Autodesk Inventor part; units mm, degrees
ref_plane "YZ Plane" through (0, 0, 0) normal (1, 0, 0) x (0, 1, 0)
ref_plane "XZ Plane" through (0, 0, 0) normal (0, 1, 0) x (-1, 0, 0)
ref_plane "XY Plane" through (0, 0, 0) normal (0, 0, 1) x (1, 0, 0)
sketch "Sketch1" plane through (0, 0, 0) normal (0, 0, 1) x (1, 0, 0)
  line L0 (0, 31.071) -> (22.7086, 31.071)
  line L1 (0, 31.071) -> (-22.7086, 31.071)
  line L2 (0, -32.929) -> (19.9189, -32.929)
  line L3 (0, -32.929) -> (-19.9189, -32.929)
  arc A0 (-22.7086, 31.071) -> (-19.9189, -32.929) centre (0, 0) ccw
  arc A1 (19.9189, -32.929) -> (22.7086, 31.071) centre (0, 0) ccw
  dimension "d2" = 64
extrude "Extrusion1" add sketch "Sketch1" along normal blind 3
properties part number "superior"
Input: part model. Units: mm. Frame: model coordinates. Give positions to 0.01 mm unless a question says otherwise; leave off trailing zeros. Write each loop counter-clockwise with the first axis right and the second up, starting at its lowest first coordinate (ties: lowest second). Pieces come first, ordered by that corner, then holes. Notation, with made-up numbers: (71.5, 39) - (113.5, 39) arc R22 cw to (113.5, 72) - close; hole circle Ø2 at (29.5, 89.5). An arc over 180 degrees is marked (long way). Write item = value, one per line. Start each with the question number.
1) Material intervals for L1, parallel to X at y = 1, z = 0.4; L2, parallel to X at y = 27.5, z = 2; L3, parallel to Y at x = 24.5, z = 1.95, sorted ascending. Write a range as [from, to].
2) Pin query (flat end, axial travel): pin 1 (6 mm diameter, centred on x = 13, y = -3.5, fed in from -Z). Return the tip coordinate at first contact, or that it passes through.
3) Cut plane B-B (y = 9). Return loops of the section in (x, z), and give its area (3 significant figures).
4) Cut plane A-A (z = 1.4). Return loops of the section in (x, y).
Answers follow:
q1.L1 = [-38.47, 38.47]
q1.L2 = [-26.92, 26.92]
q1.L3 = [-29.68, 29.68]
q2.pin_1 = 0
q3.outline = (-37.42, 0) - (37.42, 0) - (37.42, 3) - (-37.42, 3) - close
q3.area = 225 mm^2
q4.outline = (-22.71, 31.07) arc R38.48 ccw to (-19.92, -32.93) - (19.92, -32.93) arc R38.48 ccw to (22.71, 31.07) - close
